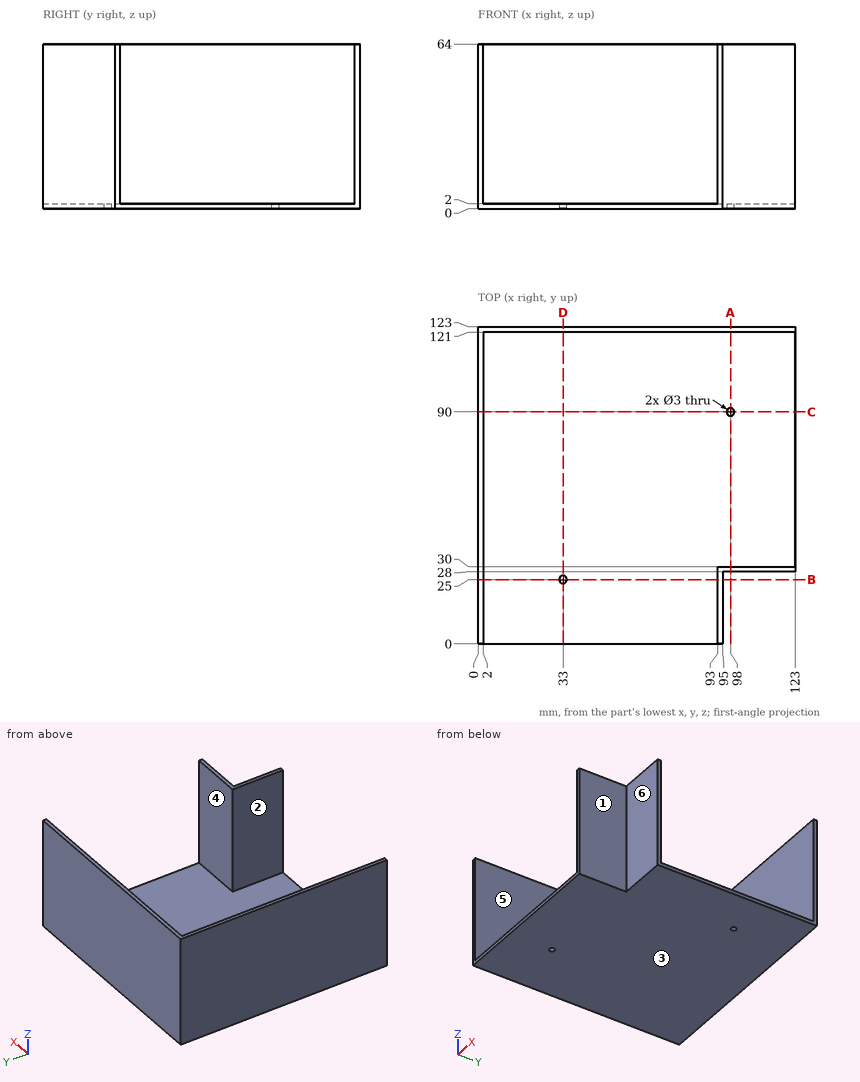
Here's the drawing with two shaded views (mm, measured from the low corner). I have some questions. A direction names the side the tool comes from. Round coordinates to 2 decimals unless told otherwise and drop trailing zeros. Loops run counter-clockwise (first coordinate to the right, second up) from the corner with the lowest first, then second, coordinate; pieces in that order, holes last. Notation, with made-up numbers: M 32.25,84.25 L 40.25,84.25 A19 ccw 40.25,100.25 Z; hole C -29.5,1.5 d8. An arc over 180 degrees is marked long. Answer as CSV lines item,"result".
1) We'd pull the mould along X, two halves only. Please class the marked faces 1, 2 and 3: released by +X, released by -X, zero draft, split by the parting line, or undercut.
From the geometry:
face 1,"released by +X"
face 2,"undercut"
face 3,"zero draft"
2) If I drill on probe 1 along Y at (x, z) = (113, 5); probe 2 along X at (y, z) = (90, 1.4); probe 3 along Y at (x, z) = (98, 1), over which ranges is the centre line in solid material (lowest first)?
From the geometry:
probe 1,"28 to 30, 121 to 123"
probe 2,"0 to 96.5, 99.5 to 123"
probe 3,"28 to 88.5, 91.5 to 123"
3) Imagine slicing it at C-C on y = 90. List the corners of the cut face in (x, z) for me, and give its area (3 significant figures).
From the geometry:
outline,"M 0,0 L 96.5,0 L 96.5,2 L 2,2 L 2,64 L 0,64 Z; M 99.5,0 L 123,0 L 123,2 L 99.5,2 Z"
area,"364 mm^2"
4) Imagine slicing it at B-B on y = 25. List the corners of the cut face in (x, z) for me.
From the geometry:
outline,"M 0,0 L 31.5,0 L 31.5,2 L 2,2 L 2,64 L 0,64 Z; M 34.5,0 L 95,0 L 95,64 L 93,64 L 93,2 L 34.5,2 Z"
5) Imagine slicing it at D-D on x = 33. List the corners of the cut face in (y, z) for me.
From the geometry:
outline,"M 0,0 L 23.5,0 L 23.5,2 L 0,2 Z; M 26.5,0 L 123,0 L 123,64 L 121,64 L 121,2 L 26.5,2 Z"
6) Imagine slicing it at A-A on x = 98. List the corners of the cut face in (y, z) for me.
From the geometry:
outline,"M 28,0 L 88.5,0 L 88.5,2 L 30,2 L 30,64 L 28,64 Z; M 91.5,0 L 123,0 L 123,64 L 121,64 L 121,2 L 91.5,2 Z"
7) For pin 1 Ø2 at (x, z) = (86, 32.5) entering from -Y; pin 2 Ø10 at (x, y) = (34.5, 48.5) entering from +Z; pin 3 Ø22.5 at (y, z) = (14.5, 28.5) entering from +X, each with a flat end and sliding along its axis, tell me the tip position at first contact or that it passes through.
From the geometry:
pin 1,"y = 121"
pin 2,"z = 2"
pin 3,"x = 95"
8) Which directions (+Z, -Z, +X, -X, +Y, -Y) give clear straight access to the entire face, cutting with the end or side of a thin tool? Please do the marked faces 4, 5 and 6.
From the geometry:
face 4,"+Z, +X"
face 5,"+Z, -Y"
face 6,"+Z, -Z, +X, -Y"
